For this review, take the finished solid that the model builds, in its own axes (mm). Give positions to 0.01 mm unless a question says otherwise; leave off trailing zeros. Write each loop counter-clockwise with the first axis right and the second up, starting at its lowest first coordinate (ties: lowest second). Pieces come first, ordered by that corner, then holes. Notation, with made-up numbers: M 30.25,41.25 L 63.25,41.25 A13 cw 63.25,64.25 Z; hole C 34.5,-16 d5. An arc over 180 degrees is marked long. One line per item, written item: value. Start each with the question number.
Item 1: Consider section C-C, the plane x = -43.15. Write out the cut boundary in (y, z), and give its area (3 significant figures).
Item 2: Consider section B-B, the plane y = 1.45. Give the number of separate pieces and of enclosed holes in the cut face, and give its area (3 significant figures).
Item 3: Consider section A-A, the plane z = 29.15. Write out the cut boundary in (x, y), and give its area (3 significant figures).
Item 4: To check wall thickness, follow probe 1 along X at (y, z) = (2.8, -29.15); probe 2 along X at (y, z) = (2.4, 35); probe 3 along Z at (x, y) = (80, 1.6). State the ranges of each line that lie inside material, in increasing order.
Item 5: Mouldability with a two-part tool opening along Z and no side actions: class faces 1 (the face through (-1, 4, -1)), 2 (the face through (-1, 2, 45)), 3 (the face through (44.367, 2.028, -27.563)) as released by +Z, released by -Z, zero draft, split by the parting line, or undercut.
```python
from build123d import *

# Parameters (mm, degrees)
CROQUIS2_W              = 180
CROQUIS2_H              = 90
SALIENTE_EXTRUIR1_DEPTH = 4
REDONDEO1_R             = 10
CORTAR_EXTRUIR2_REACH   = 102.703
CROQUIS4_R              = 4
CORTAR_EXTRUIR3_REACH   = 102.703
CROQUIS5_R              = 2


with BuildPart() as part:
    # Croquis2 → Saliente-Extruir1 (new body)
    with BuildSketch(Plane(origin=(0, 0, 0), x_dir=(1, 0, 0), z_dir=(0, 1, 0))):
        Rectangle(CROQUIS2_W, CROQUIS2_H)
    extrude(amount=SALIENTE_EXTRUIR1_DEPTH)

    # Redondeo1
    redondeo1_edges = [part.edges().sort_by_distance(p)[0] for p in [
        (90, 2, 45),
        (-90, 2, 45),
        (-90, 2, -45),
        (90, 2, -45),
    ]]
    fillet(redondeo1_edges, radius=REDONDEO1_R)

    # Croquis4 → Cortar-Extruir2 (cut, up to next)
    with BuildSketch(Plane(origin=(0, 4, 0), x_dir=(1, 0, 0), z_dir=(0, 1, 0)), mode=Mode.PRIVATE) as cortar_extruir2_sk1:
        with Locations(Location((-80, 35, 0), (0, 0, 270))):
            Circle(CROQUIS4_R)
    cortar_extruir2_tool1 = extrude(cortar_extruir2_sk1.sketch, amount=-CORTAR_EXTRUIR2_REACH, mode=Mode.PRIVATE) & part.part
    # Croquis4 → Cortar-Extruir2 (cut, up to next)
    with BuildSketch(Plane(origin=(0, 4, 0), x_dir=(1, 0, 0), z_dir=(0, 1, 0)), mode=Mode.PRIVATE) as cortar_extruir2_sk2:
        with Locations(Location((-80, -35, 0), (0, 0, 270))):
            Circle(CROQUIS4_R)
    cortar_extruir2_tool2 = extrude(cortar_extruir2_sk2.sketch, amount=-CORTAR_EXTRUIR2_REACH, mode=Mode.PRIVATE) & part.part
    # Croquis4 → Cortar-Extruir2 (cut, up to next)
    with BuildSketch(Plane(origin=(0, 4, 0), x_dir=(1, 0, 0), z_dir=(0, 1, 0)), mode=Mode.PRIVATE) as cortar_extruir2_sk3:
        with Locations(Location((80, -35, 0), (0, 0, 90))):
            Circle(CROQUIS4_R)
    cortar_extruir2_tool3 = extrude(cortar_extruir2_sk3.sketch, amount=-CORTAR_EXTRUIR2_REACH, mode=Mode.PRIVATE) & part.part
    # Croquis4 → Cortar-Extruir2 (cut, up to next)
    with BuildSketch(Plane(origin=(0, 4, 0), x_dir=(1, 0, 0), z_dir=(0, 1, 0)), mode=Mode.PRIVATE) as cortar_extruir2_sk4:
        with Locations(Location((80, 35, 0), (0, 0, 90))):
            Circle(CROQUIS4_R)
    cortar_extruir2_tool4 = extrude(cortar_extruir2_sk4.sketch, amount=-CORTAR_EXTRUIR2_REACH, mode=Mode.PRIVATE) & part.part
    add(cortar_extruir2_tool1.solids().sort_by_distance((-80, 4, -35))[0], mode=Mode.SUBTRACT)
    add(cortar_extruir2_tool2.solids().sort_by_distance((-80, 4, 35))[0], mode=Mode.SUBTRACT)
    add(cortar_extruir2_tool3.solids().sort_by_distance((80, 4, 35))[0], mode=Mode.SUBTRACT)
    add(cortar_extruir2_tool4.solids().sort_by_distance((80, 4, -35))[0], mode=Mode.SUBTRACT)

    # Croquis5 → Cortar-Extruir3 (cut, up to next)
    with BuildSketch(Plane(origin=(0, 4, 0), x_dir=(1, 0, 0), z_dir=(0, 1, 0)), mode=Mode.PRIVATE) as cortar_extruir3_sk1:
        with Locations(Location((-43.15, 29.15, 0), (0, 0, 270))):
            Circle(CROQUIS5_R)
    cortar_extruir3_tool1 = extrude(cortar_extruir3_sk1.sketch, amount=-CORTAR_EXTRUIR3_REACH, mode=Mode.PRIVATE) & part.part
    # Croquis5 → Cortar-Extruir3 (cut, up to next)
    with BuildSketch(Plane(origin=(0, 4, 0), x_dir=(1, 0, 0), z_dir=(0, 1, 0)), mode=Mode.PRIVATE) as cortar_extruir3_sk2:
        with Locations(Location((-43.15, -29.15, 0), (0, 0, 270))):
            Circle(CROQUIS5_R)
    cortar_extruir3_tool2 = extrude(cortar_extruir3_sk2.sketch, amount=-CORTAR_EXTRUIR3_REACH, mode=Mode.PRIVATE) & part.part
    # Croquis5 → Cortar-Extruir3 (cut, up to next)
    with BuildSketch(Plane(origin=(0, 4, 0), x_dir=(1, 0, 0), z_dir=(0, 1, 0)), mode=Mode.PRIVATE) as cortar_extruir3_sk3:
        with Locations(Location((43.15, -29.15, 0), (0, 0, 90))):
            Circle(CROQUIS5_R)
    cortar_extruir3_tool3 = extrude(cortar_extruir3_sk3.sketch, amount=-CORTAR_EXTRUIR3_REACH, mode=Mode.PRIVATE) & part.part
    # Croquis5 → Cortar-Extruir3 (cut, up to next)
    with BuildSketch(Plane(origin=(0, 4, 0), x_dir=(1, 0, 0), z_dir=(0, 1, 0)), mode=Mode.PRIVATE) as cortar_extruir3_sk4:
        with Locations(Location((43.15, 29.15, 0), (0, 0, 90))):
            Circle(CROQUIS5_R)
    cortar_extruir3_tool4 = extrude(cortar_extruir3_sk4.sketch, amount=-CORTAR_EXTRUIR3_REACH, mode=Mode.PRIVATE) & part.part
    add(cortar_extruir3_tool1.solids().sort_by_distance((-43.15, 4, -29.15))[0], mode=Mode.SUBTRACT)
    add(cortar_extruir3_tool2.solids().sort_by_distance((-43.15, 4, 29.15))[0], mode=Mode.SUBTRACT)
    add(cortar_extruir3_tool3.solids().sort_by_distance((43.15, 4, 29.15))[0], mode=Mode.SUBTRACT)
    add(cortar_extruir3_tool4.solids().sort_by_distance((43.15, 4, -29.15))[0], mode=Mode.SUBTRACT)


solid = part.part
```
Model answer:
1. outline: M 0,-45 L 4,-45 L 4,-31.15 L 0,-31.15 Z; M 0,-27.15 L 4,-27.15 L 4,27.15 L 0,27.15 Z; M 0,31.15 L 4,31.15 L 4,45 L 0,45 Z
1. area: 328 mm2
2. separate pieces: 1
2. enclosed holes: 8
2. area: 15,900 mm2
3. outline: M -90,0 L -45.15,0 L -45.15,4 L -90,4 Z; M -41.15,0 L 41.15,0 L 41.15,4 L -41.15,4 Z; M 45.15,0 L 90,0 L 90,4 L 45.15,4 Z
3. area: 688 mm2
4. probe 1: x = -90 to -45.15, -41.15 to 41.15, 45.15 to 90
4. probe 2: x = -90 to -84, -76 to 76, 84 to 90
4. probe 3: z = -45 to -39, -31 to 31, 39 to 45
5. face 1: zero draft
5. face 2: released by +Z
5. face 3: undercut
